Could you check a few things on this model? Use its own coordinates, in mm. A direction names the side the tool comes from. Give positions to 0.01 mm unless a question says otherwise; leave off trailing zeros. Write each loop counter-clockwise with the first axis right and the second up, starting at its lowest first coordinate (ties: lowest second). Pieces come first, ordered by that corner, then holes. Notation, with made-up numbers: M 5,48 L 24,48 A27 cw 24,79 Z; hole C 41.5,22 d6. An arc over 180 degrees is marked long. Answer as a JSON object with one key per item and string values. Group by question number.
```python
from build123d import *

# Parameters (mm, degrees)
SKETCH1_W                = 609.6
SKETCH1_H                = 457.2
BOSS_EXTRUDE1_DEPTH      = 127
SKETCH2_R                = 50.8
SKETCH2_R_2              = 25.4
BOSS_EXTRUDE2_DEPTH      = 127
BOSS_EXTRUDE3_START      = -127
SKETCH3_R                = 25.4
BOSS_EXTRUDE3_DEPTH      = 127
BOSS_EXTRUDE4_DEPTH      = 50.8
BOSS_EXTRUDE4_DEPTH_BACK = 508
SKETCH5_R                = 25.4
SKETCH6_R                = 12.7
CUT_EXTRUDE1_DEPTH       = 486.266318633
CUT_EXTRUDE2_DEPTH       = 101.6
SKETCH8_R                = 25.4
BOSS_EXTRUDE5_DEPTH      = 101.6
BOSS_EXTRUDE6_START      = 101.6
SKETCH9_R                = 25.4
BOSS_EXTRUDE6_DEPTH      = 101.6


with BuildPart() as part:
    # Sketch1 → Boss-Extrude1 (new body)
    with BuildSketch(Plane(origin=(0, 0, 0), x_dir=(1, 0, 0), z_dir=(0, 1, 0))):
        Rectangle(SKETCH1_W, SKETCH1_H)
    extrude(amount=BOSS_EXTRUDE1_DEPTH)

    # Sketch2 → Boss-Extrude2 (add)
    # profile 1 of 4: a face of its own
    with BuildSketch(Plane.XY.offset(228.6)):
        with BuildLine():
            Line((-203.2, -76.2), (-203.2, 0))
            Line((-203.2, 0), (-304.8, 0))
            Line((-304.8, 0), (-304.8, -76.2))
            ThreePointArc((-304.8, -76.2), (-254, -25.4), (-203.2, -76.2))
        make_face()
    # profile 2 of 4: a face of its own
    with BuildSketch(Plane.XY.offset(228.6)):
        with Locations((-254, -76.2)):
            Circle(SKETCH2_R)
        with Locations((-254, -76.2)):
            Circle(SKETCH2_R_2, mode=Mode.SUBTRACT)
    # profile 3 of 4: a face of its own
    with BuildSketch(Plane.XY.offset(228.6)):
        with Locations((254, -76.2)):
            Circle(SKETCH2_R)
        with Locations((254, -76.2)):
            Circle(SKETCH2_R_2, mode=Mode.SUBTRACT)
    # profile 4 of 4: a face of its own
    with BuildSketch(Plane.XY.offset(228.6)):
        with BuildLine():
            Line((304.8, -76.2), (304.8, 0))
            Line((304.8, 0), (203.2, 0))
            Line((203.2, 0), (203.2, -76.2))
            ThreePointArc((203.2, -76.2), (254, -25.4), (304.8, -76.2))
        make_face()
    extrude(amount=-BOSS_EXTRUDE2_DEPTH)

    # Sketch3 → Boss-Extrude3 (add)
    # profile 1 of 2: a face of its own
    with BuildSketch(Plane(origin=(0, 0, -228.6), x_dir=(-1, 0, 0), z_dir=(0, 0, -1)).offset(BOSS_EXTRUDE3_START)):
        with BuildLine():
            Line((-203.2, -76.2), (-203.2, 0))
            Line((-203.2, 0), (-304.8, 0))
            Line((-304.8, 0), (-304.8, -76.2))
            ThreePointArc((-304.8, -76.2), (-254, -127), (-203.2, -76.2))
        make_face()
        with Locations(Location((-254, -76.2, 0), (0, 0, 180))):
            Circle(SKETCH3_R, mode=Mode.SUBTRACT)
    # profile 2 of 2: a face of its own
    with BuildSketch(Plane(origin=(0, 0, -228.6), x_dir=(-1, 0, 0), z_dir=(0, 0, -1)).offset(BOSS_EXTRUDE3_START)):
        with BuildLine():
            Line((304.8, -76.2), (304.8, 0))
            Line((304.8, 0), (203.2, 0))
            Line((203.2, 0), (203.2, -76.2))
            ThreePointArc((203.2, -76.2), (254, -127), (304.8, -76.2))
        make_face()
        with Locations(Location((254, -76.2, 0), (0, 0, 180))):
            Circle(SKETCH3_R, mode=Mode.SUBTRACT)
    extrude(amount=BOSS_EXTRUDE3_DEPTH)

    # Sketch5 → Boss-Extrude4 (add, two sides: drawn at the far end of the back side and taken through both)
    with BuildSketch(Plane.XY.offset(228.6).offset(-BOSS_EXTRUDE4_DEPTH_BACK)):
        with Locations((254, -76.2)):
            Circle(SKETCH5_R)
        with Locations((-254, -76.2)):
            Circle(SKETCH5_R)
    extrude(amount=BOSS_EXTRUDE4_DEPTH + BOSS_EXTRUDE4_DEPTH_BACK)

    # Sketch6 → Cut-Extrude1 (cut, through all)
    with BuildSketch(Plane(origin=(0, 127, 0), x_dir=(1, 0, 0), z_dir=(0, 1, 0))):
        with Locations(Location((254, -254, 0), (0, 0, 270))):
            Circle(SKETCH6_R)
        with Locations(Location((254, 254, 0), (0, 0, 270))):
            Circle(SKETCH6_R)
    extrude(amount=-CUT_EXTRUDE1_DEPTH, mode=Mode.SUBTRACT)

    # Sketch7 → Cut-Extrude2 (cut)
    with BuildSketch(Plane(origin=(304.8, 0, 0), x_dir=(0, 0, -1), z_dir=(1, 0, 0))):
        Polygon((-228.6, -63.5), (-330.2, -63.5), (-330.2, -88.9), (-228.6, -88.9), (-228.6, -76.2), align=None)
        Polygon((279.4, -88.9), (279.4, -63.5), (228.6, -63.5), (228.6, -76.2), (228.6, -88.9), align=None)
    extrude(amount=-CUT_EXTRUDE2_DEPTH, mode=Mode.SUBTRACT)

    # Sketch8 → Boss-Extrude5 (add)
    with BuildSketch(Plane(origin=(0, 0, -279.4), x_dir=(-1, 0, 0), z_dir=(0, 0, -1))):
        with Locations(Location((254, -76.2, 0), (0, 0, 180))):
            Circle(SKETCH8_R)
    extrude(amount=BOSS_EXTRUDE5_DEPTH)

    # Sketch9 → Boss-Extrude6 (add)
    with BuildSketch(Plane.XY.offset(279.4).offset(BOSS_EXTRUDE6_START)):
        with Locations((-254, -76.2)):
            Circle(SKETCH9_R)
    extrude(amount=-BOSS_EXTRUDE6_DEPTH)


solid = part.part
```
1) For faces 4 (the flat face through (259, -88.9, -242)), 5 (the cylindrical face through (242.27, -98.73, -260)), 6 (the cylindrical face through (-272.72, -93.37, -303.73)), which set-ups out of +Z, -Z, +X, -X, +Y, -Y let a thin tool reach every point of the face, with its end or its side?
2) If we section it at A-A, the plane y = -17: List the corners of the cut face in (x, z) for me.
3) Please list where these lines run through material, in increasing order: line 1 along Z through (x, y) = (254, -92.5); line 2 along X through (y, z) = (-41.5, -138); line 3 along X through (y, z) = (-62.5, -243). Write a range as from..to.
4) If we section it at C-C, the plane x = -254: List the corners of the cut face in (y, z) for me, plus the area to 3 significant figures.
5) If we section it at D-D, the plane y = 91: List the corners of the cut face in (x, z) for me.
6) We'd pull the mould along X, two halves only. Please class faces 1 (the flat face through (259, -63.5, -266)), 2 (the cylindrical face through (-255.117, -126.988, 165.989)), 3 (the cylindrical face through (249.136, -93.75, 265.732)): released by +X, released by -X, zero draft, split by the parting line, or undercut.
7) I'm going to push flat-ended pins straight in: pin 1 (10 mm diameter, centred on x = 5, y = 69, fed in from +Z); pin 2 (2 mm diameter, centred on x = 94.5, y = 15, fed in from -Z); pin 3 (4 mm diameter, centred on x = 248.5, y = -93.5, fed in from -Z). Where does each tip first touch, or does it pass through?
8) If we section it at B-B, the plane z = 217.5: List the corners of the cut face in (x, y) for me.
Taken from the geometry:
{
 "1": {"face 4": "-Z, +X", "face 5": "-Z, -Y", "face 6": "-Z"},
 "2": {"outline": "M -304.8,-228.6 L -203.2,-228.6 L -203.2,-101.6 L -304.8,-101.6 Z; M -304.8,101.6 L -203.2,101.6 L -203.2,228.6 L -304.8,228.6 Z; M 203.2,-228.6 L 304.8,-228.6 L 304.8,-101.6 L 203.2,-101.6 Z; M 203.2,101.6 L 304.8,101.6 L 304.8,228.6 L 203.2,228.6 Z"},
 "3": {"line 1": "-279.4..-266.7, -241.3..241.3, 266.7..279.4", "line 2": "-304.8..-203.2, 203.2..304.8", "line 3": "-275.39..-232.61, 232.61..247.65, 260.35..275.39"},
 "4": {"outline": "M -127,-228.6 L -101.6,-228.6 L -101.6,-381 L -50.8,-381 L -50.8,-228.6 L 127,-228.6 L 127,228.6 L -50.8,228.6 L -50.8,381 L -101.6,381 L -101.6,228.6 L -127,228.6 L -127,101.6 L -101.6,101.6 L -101.6,-101.6 L -127,-101.6 Z; hole M -50.8,-101.6 L 0,-101.6 L 0,101.6 L -50.8,101.6 Z", "area": "116,000 mm²"},
 "5": {"outline": "M -304.8,-228.6 L 304.8,-228.6 L 304.8,228.6 L -304.8,228.6 Z"},
 "6": {"face 1": "zero draft", "face 2": "undercut", "face 3": "undercut"},
 "7": {"pin 1": "z = 228.6", "pin 2": "z = -228.6", "pin 3": "z = -279.4"},
 "8": {"outline": "M -304.8,-76.2 A50.8 ccw -203.2,-76.2 L -203.2,0 L 203.2,0 L 203.2,-76.2 A50.8 ccw 304.8,-76.2 L 304.8,127 L -304.8,127 Z"}
}
